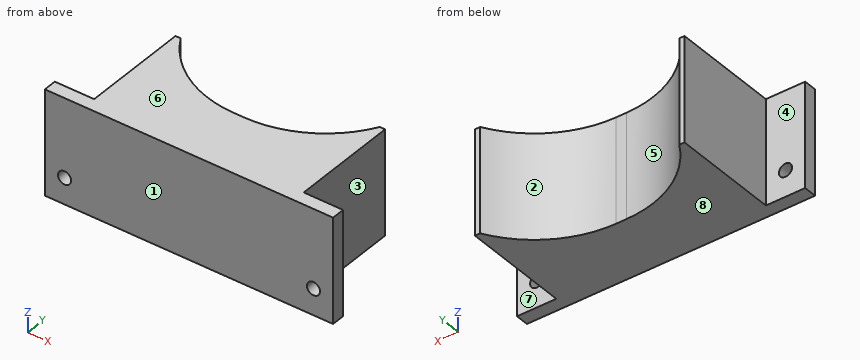
from build123d import *

# Parameters (mm, degrees)
BOSS_EXTRUDE1_DEPTH = 40
SKETCH3_R           = 2.5
CUT_EXTRUDE1_DEPTH  = 40


with BuildPart() as part:
    # Sketch1 → Boss-Extrude1 (new body)
    with BuildSketch(Plane.XY):
        with BuildLine():
            Line((55, 0), (-55, 0))
            Line((-55, 0), (-55, 5))
            Line((-55, 5), (-40, 5))
            Line((-40, 5), (-40, 46))
            Line((-40, 46), (-38, 46))
            ThreePointArc((-38, 46), (-22.838665984, 30.633715456), (-2, 25))
            Line((-2, 25), (2, 25))
            ThreePointArc((2, 25), (22.838665984, 30.633715456), (38, 46))
            Line((38, 46), (40, 46))
            Line((40, 46), (40, 5))
            Line((40, 5), (55, 5))
            Line((55, 5), (55, 0))
        make_face()
    extrude(amount=BOSS_EXTRUDE1_DEPTH)

    # Sketch3 → Cut-Extrude1 (cut)
    with BuildSketch(Plane(origin=(0, 5, 0), x_dir=(1, 0, 0), z_dir=(0, 1, 0))):
        with Locations((-47.5, -10)):
            Circle(SKETCH3_R)
        with Locations((47.5, -10)):
            Circle(SKETCH3_R)
    extrude(amount=-CUT_EXTRUDE1_DEPTH, mode=Mode.SUBTRACT)


solid = part.part
Input: part model. Units: mm. Frame: model coordinates. Face numbers are marked on the shaded views. A direction names the side the tool comes from. Coordinates: 2 decimals unless noted, no trailing zeros. Loops run counter-clockwise (first coordinate to the right, second up) from the corner with the lowest first, then second, coordinate; pieces in that order, holes last. Notation, with made-up numbers: (-31.5, 61) -> (-15.5, 61) arc R12 cw to (-15.5, 73) -> close; hole circle Ø4 at (8, 60). An arc over 180 degrees is marked (long way). One line per item, written item: value.
(1) Cut plane A-A (z = 10). Output: boundary loops of the cut face in (x, y), then the cut area to 3 significant figures.
Answer below:
outline: (-55, 0) -> (-50, 0) -> (-50, 5) -> (-55, 5) -> close; (-45, 0) -> (45, 0) -> (45, 5) -> (40, 5) -> (40, 46) -> (38, 46) arc R41.36 cw to (2, 25) -> (-2, 25) arc R41.36 cw to (-38, 46) -> (-40, 46) -> (-40, 5) -> (-45, 5) -> close; (50, 0) -> (55, 0) -> (55, 5) -> (50, 5) -> close
area: 2,620 mm2
(2) Ray query, line 1 along X through (y, z) = (3, 10); line 2 along Z through (x, y) = (-47.5, 3.85); line 3 along X through (y, z) = (22, 25.5). Return the intervals inside material, ascending.
Answer below:
line 1: x = -55 to -50, -45 to 45, 50 to 55
line 2: z = 0 to 7.5, 12.5 to 40
line 3: x = -40 to 40
(3) Set-up query: the marked faces 4, 5, 6, 7 and 8. Return all of +Z, -Z, +X, -X, +Y, -Y with unobstructed straight access to the full face (end or side cutting, diameter ignored); none if empty.
Answer below:
face 4: +Z, -Z, -X, +Y
face 5: +Z, -Z, +Y
face 6: +Z, +X, -X, +Y, -Y
face 7: +Z, -Z, +X, +Y
face 8: -Z, +X, -X, +Y, -Y
(4) Pin query (flat end, axial travel): pin 1 Ø7.5 at (x, z) = (-47, 23.5) entering from +Y; pin 2 Ø8 at (y, z) = (10.5, 18) entering from +X; pin 3 Ø12 at (y, z) = (17, 28.5) entering from -X. Return the tip coordinate at first contact, or that it passes through.
Answer below:
pin 1: stops at y = 5
pin 2: stops at x = 40
pin 3: stops at x = -40
(5) Cut plane C-C (y = 34). Output: boundary loops of the cut face in (x, z), then the cut area to 3 significant figures.
Answer below:
outline: (-40, 0) -> (-27.76, 0) -> (-27.76, 40) -> (-40, 40) -> close; (27.76, 0) -> (40, 0) -> (40, 40) -> (27.76, 40) -> close
area: 979 mm2
(6) Draft query along Y for the marked faces 1, 2 and 3. Return one class per face: pulls with the +Y half, pulls with the -Y half, needs draft (parallel to the pull), parting line crosses it, or undercut.
Answer below:
face 1: pulls with the -Y half
face 2: pulls with the +Y half
face 3: needs draft
(7) Cut plane B-B (x = 47.5). Output: boundary loops of the cut face in (y, z).
Answer below:
outline: (0, 0) -> (5, 0) -> (5, 7.5) -> (0, 7.5) -> close; (0, 12.5) -> (5, 12.5) -> (5, 40) -> (0, 40) -> close
(8) Cut plane D-D (z = 24). Output: boundary loops of the cut face in (x, y), then the cut area to 3 significant figures.
Answer below:
outline: (-55, 0) -> (55, 0) -> (55, 5) -> (40, 5) -> (40, 46) -> (38, 46) arc R41.36 cw to (2, 25) -> (-2, 25) arc R41.36 cw to (-38, 46) -> (-40, 46) -> (-40, 5) -> (-55, 5) -> close
area: 2,670 mm2
